Read the model definition and answer for the solid it produces. Units are mm, in the model's axes. A direction names the side the tool comes from. Coordinates: 2 decimals unless noted, no trailing zeros. Order: outer loops, then holes, each group sorted by start corner. A loop starts at its lowest first (then second) coordinate and runs counter-clockwise, first axis right, second up. Notation, with made-up numbers: (89.25, 43) - (129.25, 43) arc R26 cw to (129.25, 59) - close; hole circle Ø1 at (71.25, 9). An arc over 180 degrees is marked (long way). Use one line per item in the form item = value.
```python
from build123d import *

# Parameters (mm, degrees)
F1_DEPTH = 1
F3_DEPTH = 12
F5_DEPTH = 1


with BuildPart() as f1:
    # F0 (on Top) → F1 (new body)
    with BuildSketch(Plane.XY):
        Polygon((-115, -42.5), (115, -42.5), (115, 42.5), (-57, 42.5), (-115, -15.5), align=None)
    extrude(amount=F1_DEPTH)

    # F2 (on face) → F3 (join)
    with BuildSketch(Plane.XY.offset(1)):
        Polygon((-115, -15.5), (-115, -42.5), (-114, -42.5), (-114, -15.9142135624), (-56.5857864376, 41.5), (114, 41.5), (114, -42.5), (115, -42.5), (115, 42.5), (-57, 42.5), align=None)
    extrude(amount=F3_DEPTH)

    # F4 (on face) → F5 (cut)
    with BuildSketch(Plane(origin=(-49.75, 49.75, 0), x_dir=(-0.7071067812, -0.7071067812, 0), z_dir=(-0.7071067812, 0.7071067812, 0))):
        Polygon((92.2674349448, 0), (92.2774349448, 0), (92.2774349448, 13), (79.2674349448, 13), align=None)
        Polygon((23.3530483272, 13), (10.2530483272, 13), (10.2530483272, 0), (10.3530483272, 0), align=None)
    extrude(amount=-F5_DEPTH, mode=Mode.SUBTRACT)


solid = f1.part
```
(1) Given pin 1 Ø2 at (y, z) = (32, 6.5) entering from -X; pin 2 Ø4 at (x, z) = (82, 9) entering from -Y; pin 3 Ø2 at (x, y) = (-52.5, 5) entering from +Z; pin 4 Ø1 at (x, y) = (77.5, 21) entering from -Z, each flat-ended and moving along its own axis, determine where each tip first touches the part or whether it passes through.
Answer list:
pin_1 = -68.5
pin_2 = 41.5
pin_3 = 1
pin_4 = 0
(2) Section C-C, the plane x = -16 is taken. Write down the section's boundary in (y, z), then the cut area to 3 significant figures.
Answer list:
outline = (-42.5, 0) - (42.5, 0) - (42.5, 13) - (41.5, 13) - (41.5, 1) - (-42.5, 1) - close
area = 97.0 mm2
(3) Section D-D, the plane y = 7.5 is taken. Write down the section's boundary in (x, z), then the cut area to 3 significant figures.
Answer list:
outline = (-92, 0) - (115, 0) - (115, 13) - (114, 13) - (114, 1) - (-90.59, 1) - (-90.59, 13) - (-92, 13) - close
area = 236 mm2
(4) Which of the six approach directions +Z, -Z, +X, -X, +Y, -Y give full straight-line access (tool end or side, diameter ignored) to faces 4 (the flat face through (-2, 0, 1)), 5 (the flat face through (-2, 1, 0))?
Answer list:
face_4 = +Z, -Y
face_5 = -Z, +X, -X, +Y, -Y
(5) Straight lines are drawn through the part: L1, parallel to X at y = -25.5, z = 1.75; L2, parallel to Z at x = -49, y = -16; L3, parallel to Y at x = 15, z = 6.5. For each, find the intervals that lie inside material, in ascending order.
Answer list:
L1 = -115 to -114, 114 to 115
L2 = 0 to 1
L3 = 41.5 to 42.5
(6) Section B-B, the plane y = -28 is taken. Write down the section's boundary in (x, z).
Answer list:
outline = (-115, 0) - (115, 0) - (115, 13) - (114, 13) - (114, 1) - (-114, 1) - (-114, 13) - (-115, 13) - close
(7) Section A-A, the plane z = 6.5 is taken. Write down the section's boundary in (x, y), then the cut area to 3 significant figures.
Answer list:
outline = (-115, -42.5) - (-114, -42.5) - (-114, -15.91) - (-114.29, -16.21) - (-115, -15.5) - close; (-110.4, -10.9) - (-109.69, -11.6) - (-60.96, 37.13) - (-61.67, 37.83) - close; (-57, 42.5) - (-56.29, 41.79) - (-56.59, 41.5) - (114, 41.5) - (114, -42.5) - (115, -42.5) - (115, 42.5) - close
area = 351 mm2
(8) The mould has two halves that part along X. Classify faces 1 (the flat face through (-85.6, 13.9, 6.4)), 2 (the flat face through (114, 0, 7)), 3 (the flat face through (-86, 13, 13)): +X half, -X half, draft (parallel to the pull), parting line (faces both ways), or undercut.
Answer list:
face_1 = -X half
face_2 = undercut
face_3 = draft
